Input: part model. Units: mm. Frame: model coordinates. A direction names the side the tool comes from. Coordinates: 2 decimals unless noted, no trailing zeros. Write each loop counter-clockwise with the first axis right and the second up, starting at its lowest first coordinate (ties: lowest second). Pieces come first, ordered by that corner, then holes. Notation, with made-up numbers: (82, 22.5) - (91, 22.5) arc R5 ccw to (91, 26.5) - close; hole circle Ø10 at (87.5, -13). An arc over 180 degrees is marked (long way). Use a Markdown table: item, result. Add a question column.
Q1. Mould query, pull axis Y, two halves, no side actions, for faces 1 (the face through (-47.4, 11.1, 50)), 2 (the face through (-1, 1, 2.5)), 3 (the face through (47.69, 15.02, 24.16)). Classes: released by +Y, released by -Y, zero draft, split by the parting line, or undercut.
Q2. Material intervals for probe 1 along X at (y, z) = (1, 45); probe 2 along Y at (x, z) = (0, 39); probe 3 along Z at (x, y) = (27, 21), sorted ascending. Write a range as from..to.
Q3. Section query B-B (y = 0). Return the cut outline in (x, z).
Q4. Section query A-A (z = 17). Return the cut outline in (x, y), then the cut area to 3 significant figures.
Q5. Pin query (flat end, axial travel): P1, Ø4, axis at y = -20.5, z = 22, coming from the -X side; P2, Ø2, axis at x = -3.5, z = 12.5, coming from the +Y side; P3, Ø3, axis at x = -10.5, z = 24.5, coming from the -Y side. Return the tip coordinate at first contact, or that it passes through.
Q6. Set-up query: faces 4 (the face through (-10.3, -46.37, 25.93)), 5 (the face through (-1, 1, 0)). Return all of +Z, -Z, +X, -X, +Y, -Y with unobstructed straight access to the full face (end or side cutting, diameter ignored); none if empty.
from build123d import *

# Parameters (mm, degrees)
F0_R     = 50
F1_DEPTH = 50
F2_T     = -2.5
F3_R     = 1


with BuildPart() as f1:
    # F0 (on Top) → F1 (new body)
    with BuildSketch(Plane.XY):
        Circle(F0_R)
    extrude(amount=F1_DEPTH)

    # F2
    f2_openings = [f1.faces().sort_by_distance(p)[0] for p in [
        (0, 0, 50),
    ]]
    offset(amount=F2_T, openings=f2_openings)

    # F3
    f3_edges = [f1.edges().sort_by_distance(p)[0] for p in [
        (-50, 0, 50),
        (-47.5, 0, 50),
        (-47.5, 0, 2.5),
    ]]
    fillet(f3_edges, radius=F3_R)


solid = f1.part
Values follow:
| question | item | result |
|---|---|---|
| 1 | face 1 | zero draft |
| 1 | face 2 | undercut |
| 1 | face 3 | split by the parting line |
| 2 | probe 1 | -49.99..-47.49, 47.49..49.99 |
| 2 | probe 2 | -50..-47.5, 47.5..50 |
| 2 | probe 3 | 0..2.5 |
| 3 | outline | (-50, 0) - (50, 0) - (50, 49) arc R1 ccw to (49, 50) - (48.5, 50) arc R1 ccw to (47.5, 49) - (47.5, 3.5) arc R1 cw to (46.5, 2.5) - (-46.5, 2.5) arc R1 cw to (-47.5, 3.5) - (-47.5, 49) arc R1 ccw to (-48.5, 50) - (-49, 50) arc R1 ccw to (-50, 49) - close |
| 4 | outline | circle Ø100 at (0, 0); hole circle Ø95 at (0, 0) |
| 4 | area | 766 mm2 |
| 5 | P1 | x = -46.45 |
| 5 | P2 | y = 49.94 |
| 5 | P3 | y = -49.18 |
| 6 | face 4 | +Z |
| 6 | face 5 | -Z, +X, -X, +Y, -Y |
